Geometry check sheet. Reference: the model listing, model coordinates, mm. A direction names the side the tool comes from. Round coordinates to 2 decimals unless told otherwise and drop trailing zeros. Write each loop counter-clockwise with the first axis right and the second up, starting at its lowest first coordinate (ties: lowest second). Pieces come first, ordered by that corner, then holes.
from build123d import *

# Parameters (mm, degrees)
F0_R     = 3.5
F0_R_2   = 17.5
F0_R_3   = 24
F1_DEPTH = 3


with BuildPart() as f1:
    # F0 (on Top) → F1 (new body)
    with BuildSketch(Plane.XY):
        with BuildLine():
            Line((154.276346, 9.999091), (2.315824, 10.998961))
            ThreePointArc((2.315824, 10.998961), (-37.275268, -9.405556), (-43.049419, -53.569546))
            Line((-43.049419, -53.569546), (-31.011758, -86.297638))
            ThreePointArc((-31.011758, -86.297638), (-30.101849, -92.079184), (-31.473705, -97.768843))
            Line((-31.473705, -97.768843), (-33.380198, -101.893724))
            ThreePointArc((-33.380198, -101.893724), (-34.752053, -107.583383), (-33.842145, -113.364929))
            Line((-33.842145, -113.364929), (-21.310521, -147.436013))
            ThreePointArc((-21.310521, -147.436013), (26.12288, -189.038234), (86.815639, -171.802768))
            Line((86.815639, -171.802768), (146.405169, -113.43495))
            ThreePointArc((146.405169, -113.43495), (149.706985, -108.602536), (150.908181, -102.874418))
            Line((150.908181, -102.874418), (150.938576, -99.93974))
            ThreePointArc((150.938576, -99.93974), (152.139772, -94.211622), (155.441588, -89.379208))
            Line((155.441588, -89.379208), (183.389314, -62.00447))
            ThreePointArc((183.389314, -62.00447), (192.937656, -16.256463), (154.276346, 9.999091))
        make_face()
        with Locations((-2, -142)):
            Circle(F0_R, mode=Mode.SUBTRACT)
        with Locations((76, -160)):
            Circle(F0_R, mode=Mode.SUBTRACT)
        with Locations((115, -119)):
            Circle(F0_R, mode=Mode.SUBTRACT)
        with Locations((-33, -48)):
            Circle(F0_R, mode=Mode.SUBTRACT)
        with BuildLine():
            ThreePointArc((8, -56), (40, -24), (72, -56))
            Line((72, -56), (72, -59))
            ThreePointArc((72, -59), (40, -91), (8, -59))
            Line((8, -59), (8, -56))
        make_face(mode=Mode.SUBTRACT)
        with Locations((-6.838835, -28.161165)):
            Circle(F0_R_2, mode=Mode.SUBTRACT)
        Circle(F0_R, mode=Mode.SUBTRACT)
        with Locations((181.712813, -48)):
            Circle(F0_R, mode=Mode.SUBTRACT)
        with Locations((154, -32)):
            Circle(F0_R_3, mode=Mode.SUBTRACT)
        with Locations((154, 0)):
            Circle(F0_R, mode=Mode.SUBTRACT)
    extrude(amount=F1_DEPTH)


solid = f1.part
1. Section check B-B (y = -14.5). Record the cut outline in (x, z).
2. Section check D-D (y = -142). Record the cut outline in (x, z).
3. Release check for a two-part mould opening along X. For faces 1 (the face through (157.34, 1.05, 1.48)), 2 (the face through (-27.664, -130.162, 1.479)), 3 (the face through (25.23, -188.83, 1.48)) record: +X half, -X half, draft (parallel to the pull), parting line (faces both ways), or undercut.
4. Access from +Z, -Z, +X, -X, +Y, -Y to the whole of each face (thin tool, end or side, straight path). Record for faces 4 (the face through (73, -88, 0)), 5 (the face through (40.704, -90.992, 1.479)), 6 (the face through (-37.115, -69.704, 1.479)).
5. Scan lines: line 1 along X through (y, z) = (-22, 1.85); line 2 along Y through (x, z) = (-2, 2.15); line 3 along Y through (x, z) = (51.5, 1.95). Record each from-to range of solid material in increasing order.
6. Section check A-A (x = 40). Record the cut outline in (y, z).
7. Section check C-C (z = 1.3). State how many separate pieces and enclosed holes the cut face has, plus the area to 3 significant figures.
Results below:
1. outline: (-40.4, 0) - (-17.78, 0) - (-17.78, 3) - (-40.4, 3) - close; (4.1, 0) - (137.58, 0) - (137.58, 3) - (4.1, 3) - close; (170.42, 0) - (192.18, 0) - (192.18, 3) - (170.42, 3) - close
2. outline: (-23.31, 0) - (-5.5, 0) - (-5.5, 3) - (-23.31, 3) - close; (1.5, 0) - (117.24, 0) - (117.24, 3) - (1.5, 3) - close
3. face 1: undercut
3. face 2: -X half
3. face 3: parting line
4. face 4: -Z, +X, -X, +Y, -Y
4. face 5: +Z, -Z
4. face 6: +Z, -Z, -X
5. line 1: x = -43.6 to -23.22, 9.54 to 132.18, 175.82 to 194.79
5. line 2: y = -175.04 to -145.5, -138.5 to -44.98, -11.34 to -2.87, 2.87 to 10.83
5. line 3: y = -189.75 to -88.86, -26.14 to 10.68
6. outline: (-190.65, 0) - (-91, 0) - (-91, 3) - (-190.65, 3) - close; (-24, 0) - (10.75, 0) - (10.75, 3) - (-24, 3) - close
7. separate pieces: 1
7. enclosed holes: 10
7. area: 29,400 mm2
